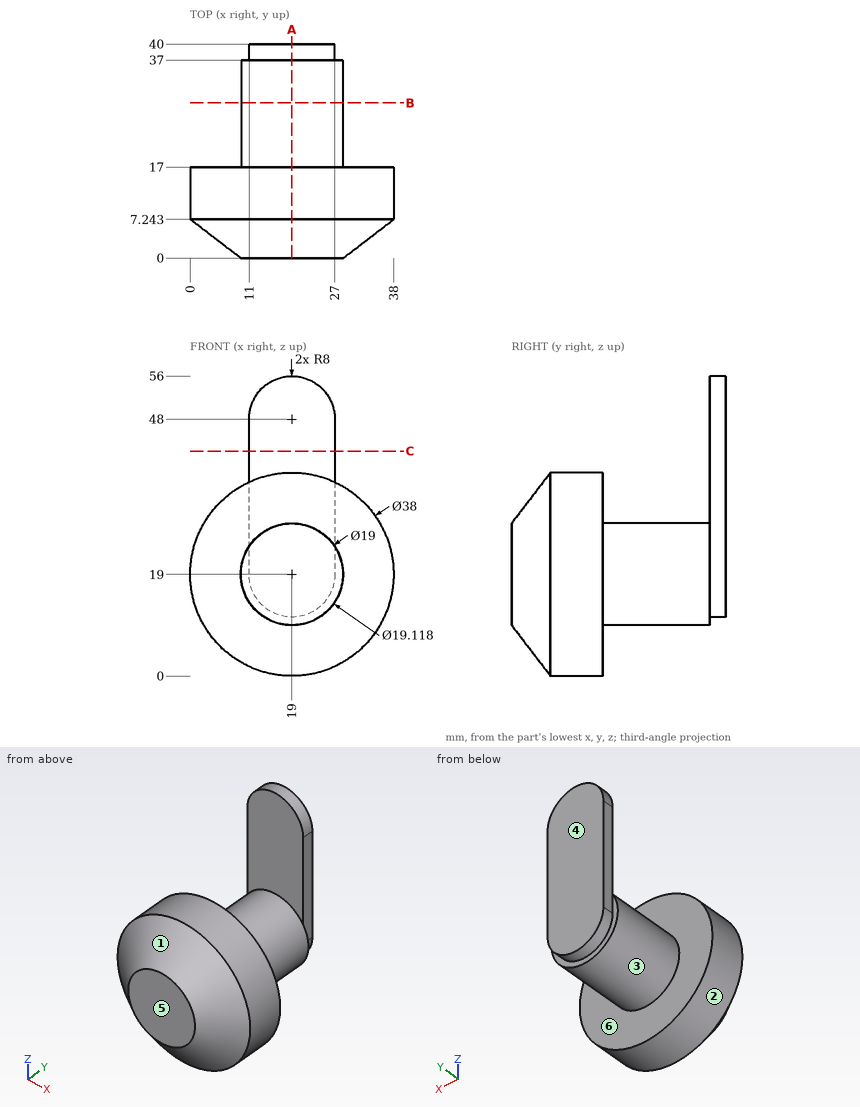
Study the drawing (mm; zero at the part's minimum x, y, z) and answer. A direction names the side the tool comes from. Coordinates: 2 decimals unless noted, no trailing zeros. Write each loop counter-clockwise with the first axis right and the second up, starting at its lowest first coordinate (ties: lowest second). Pieces come first, ordered by that corner, then holes. Notation, with made-up numbers: (18, 15.5) - (59, 15.5) arc R15 cw to (59, 35.5) - close; hole circle Ø2 at (12, -39.75). An arc over 180 degrees is marked (long way). Answer as a JSON object with one key per item and string values.
Q1. Find section B-B (y = 29). Write down the section's boundary in (x, z), plus the area to 3 significant figures.
Results list:
{"outline": "circle Ø19 at (19, 19)", "area": "284 mm^2"}
Q2. Which of the six approach directions +Z, -Z, +X, -X, +Y, -Y give full straight-line access (tool end or side, diameter ignored) to the marked faces 5 and 6?
Results list:
{"face 5": "+Z, -Z, +X, -X, -Y", "face 6": "none"}
Q3. Find section C-C (z = 42). Write down the section's boundary in (x, y), plus the area to 3 significant figures.
Results list:
{"outline": "(11, 37) - (27, 37) - (27, 40) - (11, 40) - close", "area": "48.0 mm^2"}
Q4. Consider L1, parallel to Y at x = 15, z = 53; L2, parallel to Y at x = 18, z = 30; L3, parallel to X at y = 13.5, z = 16.5 (1 decimal). Determine where each line is inside the solid, lowest interval first. Write a range as from..to.
Results list:
{"L1": "y = 37..40", "L2": "y = 1.14..17, 37..40", "L3": "x = 0.2..37.8"}
Q5. Given pin 1 Ø8 at (x, z) = (21.5, 47) entering from -Y; pin 2 Ø3 at (x, y) = (16.5, 13) entering from -Z; pin 3 Ø1.5 at (y, z) = (38, 31.5) entering from +X; pin 4 Ø2 at (y, z) = (18, 38.5) entering from -X, each flat-ended and moving along its own axis, determine where each tip first touches the part or whether it passes through.
Results list:
{"pin 1": "stops at y = 37", "pin 2": "stops at z = 0.03", "pin 3": "stops at x = 27", "pin 4": "passes through"}
Q6. For a pull along Y with two mould halves and no side action, classify the marked faces 1, 2, 3 and 4 as pulls with the +Y half, pulls with the -Y half, needs draft (parallel to the pull), parting line crosses it, or undercut.
Results list:
{"face 1": "pulls with the -Y half", "face 2": "needs draft", "face 3": "undercut", "face 4": "pulls with the +Y half"}
Q7. Find section A-A (x = 19). Write down the section's boundary in (y, z).
Results list:
{"outline": "(0, 9.44) - (7.24, 0) - (17, 0) - (17, 9.5) - (37, 9.5) - (37, 11) - (40, 11) - (40, 56) - (37, 56) - (37, 28.5) - (17, 28.5) - (17, 38) - (7.24, 38) - (0, 28.56) - close"}
